Autodesk Inventor part; units mm, degrees
ref_plane "YZ Plane" through (0, 0, 0) normal (1, 0, 0) x (0, 1, 0)
ref_plane "XZ Plane" through (0, 0, 0) normal (0, 1, 0) x (-1, 0, 0)
ref_plane "XY Plane" through (0, 0, 0) normal (0, 0, 1) x (1, 0, 0)
sketch "Sketch1" plane through (0, 0, 0) normal (0, 0, 1) x (1, 0, 0)
  circle A0 centre (0, 0) radius 15
  dimension "d0" = 30
extrude "Extrusion1" add sketch "Sketch1" along normal blind 24.5
chamfer "Chamfer1" distance 1 angle 45 2 edges at (-15, 0, 24.5) (-15, 0, 0)
sketch "Sketch2" plane through (0, 0, 24.5) normal (0, 0, 1) x (1, 0, 0)
  circle A0 centre (0, 0) radius 15
  dimension "d6" = 30
extrude "Extrusion2" add sketch "Sketch2" along normal blind 5.5
chamfer "Chamfer2" distance 1 angle 45 1 edges at (-15, 0, 24.5)
sketch "Sketch3" plane through (0, 0, 30) normal (0, 0, 1) x (1, 0, 0)
  circle A0 centre (0, 0) radius 11
  dimension "d12" = 22
extrude "Extrusion3" add sketch "Sketch3" along normal blind 4
chamfer "Chamfer3" distance 4 angle 45 1 edges at (-11, 0, 30)
sketch "Sketch4" plane through (0, 0, 34) normal (0, 0, 1) x (1, 0, 0)
  circle A0 centre (0, 0) radius 11
  dimension "d18" = 22
extrude "Extrusion4" add sketch "Sketch4" along normal blind 5
sketch "Sketch5" plane through (0, 0, 39) normal (0, 0, 1) x (1, 0, 0)
  circle A0 centre (0, 0) radius 9.5
  dimension "d21" = 19
extrude "Extrusion5" add sketch "Sketch5" along normal blind 3.8
chamfer "Chamfer4" distance 1 angle 45 1 edges at (-11, 0, 39)
sketch "Sketch6" plane through (0, 0, 42.8) normal (0, 0, 1) x (1, 0, 0)
  circle A0 centre (0, 0) radius 6.6
  dimension "d27" = 13.2
extrude "Extrusion6" add sketch "Sketch6" along normal blind 0.75
sketch "Sketch7" plane through (0, 0, 43.55) normal (0, 0, 1) x (1, 0, 0)
  circle A0 centre (0, 0) radius 3.55
  dimension "d30" = 7.1
extrude "Extrusion7" add sketch "Sketch7" along normal blind 1.25
sketch "Sketch8" plane through (0, 0, 0) normal (0, 1, 0) x (-1, 0, 0)
  line L0 (3.55, 44.8) -> (-3.55, 44.8)
  line L1 (3.55, 44.8) -> (6.6, 44.0124)
  line L2 (3.55, 44.8) -> (6.7001, 44.8) construction
  line L3 (6.6, 43.55) -> (-6.6, 43.55)
  line L4 (6.6, 44.0124) -> (6.6, 43.55)
  line L5 (6.6, 43.55) -> (3.55, 43.55)
  line L6 (3.55, 43.55) -> (3.55, 44.8)
  line L7 (3.55, 44.8) -> (3.55, 43.7812)
  line L8 (0, -8.96) -> (0, 53.76)
  point P0 (0, 0)
  dimension "d33" = 14.48
revolve "Revolution1" add sketch "Sketch8" angle 360 about axis through (0, 0, -10) along (0, 0, 1) contours L1 L4 L3 L6
sketch "Sketch9" plane through (0, 0, 44.8) normal (0, 0, 1) x (1, 0, 0)
  circle A0 centre (0, 0) radius 1
  dimension "d35" = 2
extrude "Extrusion8" cut sketch "Sketch9" against normal blind 50
sketch "Sketch10" plane through (0, 0, 0) normal (0, 0, -1) x (-1, 0, 0)
  circle A0 centre (0, 0) radius 2
  dimension "d38" = 4
extrude "Extrusion9" cut sketch "Sketch10" against normal blind 20
chamfer "Chamfer5" distance 0.5 angle 45 1 edges at (-9.5, 0, 42.8)
properties part number "210505 - Zeiss x100 objective mockup"
Geometry: final body of the model. Coordinates: model frame, mm. A direction names the side the tool comes from. Round coordinates to 2 decimals unless told otherwise and drop trailing zeros. Order: outer loops, then holes, each group sorted by start corner. A loop starts at its lowest first (then second) coordinate and runs counter-clockwise, first axis right, second up. Notation, with made-up numbers: M -22.5,30.25 L 27.5,30.25 A23 ccw 27.5,49.25 Z; hole C -7,39 d3. An arc over 180 degrees is marked long. Use one line per item in the form item = value. Start each with the question number.
Q1. Cut plane B-B (z = 29). Return loops of the section in (x, y), and give its area (3 significant figures).
Q2. Cut plane A-A (z = 13). Return loops of the section in (x, y).
Q3. Access query for faces 1 (the face through (4.38, 8.43, 40.63)), 2 (the face through (-1, -1, 20)), 3 (the face through (0, -1, 33)). Directions: +Z, -Z, +X, -X, +Y, -Y. A direction counts if a zero-diameter tool reaches every point of the face in a straight line with its end or side. Return the directions, or none.
Q4. Pin query (flat end, axial travel): pin 1 Ø15 at (x, y) = (5, 4.5) entering from +Z; pin 2 Ø5 at (y, z) = (-2.5, 36) entering from -X; pin 3 Ø1.8 at (x, y) = (0, 0) entering from +Z; pin 4 Ø1.5 at (y, z) = (-2.5, 17.5) entering from -X. Return the tip coordinate at first contact, or that it passes through.
Q5. Material intervals for line 1 (Y direction, x = 0, z = 26); line 2 (Y direction, x = 0, z = 6.5); line 3 (Z direction, x = -6, y = 8), sorted ascending. Write a range as [from, to].
Geometry results:
q1.outline = C 0,0 d30; hole C 0,0 d2
q1.area = 704 mm^2
q2.outline = C 0,0 d30; hole C 0,0 d4
q3.face_1 = +Z
q3.face_2 = -Z
q3.face_3 = +Z, -Z
q4.pin_1 = 44.8
q4.pin_2 = -11.27
q4.pin_3 = through
q4.pin_4 = -14.9
q5.line_1 = [-15, -1], [1, 15]
q5.line_2 = [-15, -2], [2, 15]
q5.line_3 = [0, 39]
